```python
from build123d import *

# Parameters (mm, degrees)
F0_R        = 4.15
F1_DEPTH    = 2
F2_SIZE     = 1.99999
F3_T1_DEPTH = 51.7493718553


# Not quite as in the source:
# - a fillet or chamfer that OpenCascade refuses, or shapes differently, is made with other operations: its cross-section is extruded or revolved along the edge and cut away or added
# - a fillet or chamfer is up to 0.001 mm smaller than in the source, because OpenCascade refuses the exact size


with BuildPart() as f1:
    # F0 (on Front) → F1 (new body)
    with BuildSketch(Plane.XZ):
        Polygon((87.85, 18), (0, 18), (0, -18), (87.85, -18), (87.85, -9), (105.35, -9), (110.85, -1.42), (110.85, 1.42), (105.35, 9), (87.85, 9), align=None)
        with Locations((12, 0)):
            Circle(F0_R, mode=Mode.SUBTRACT)
        with Locations((28.5, 0)):
            Circle(F0_R, mode=Mode.SUBTRACT)
        Polygon((91.1, 5.5), (91.1, 3), (84.35, 3), (84.35, -3), (91.1, -3), (91.1, -5.5), (81.85, -5.5), (81.85, 5.5), align=None, mode=Mode.SUBTRACT)
    extrude(amount=F1_DEPTH)

    # F2 (size 2 in the source; OpenCascade refuses exactly that, so slightly less here)
    f2_edges = [f1.edges().sort_by_distance(p)[0] for p in [
        (7.85, -2, 0),
        (24.35, -2, 0),
    ]]
    chamfer(f2_edges, length=F2_SIZE)

    # F3: fillet of radius 10 on 2 edges, made by hand

    # F3_s2 → F3_t1 (cut)
    with BuildSketch(Plane.XZ.offset(-24.8746859277)):
        with BuildLine():
            ThreePointArc((77.9001256289, 18), (84.6083295614, 15.4161984871), (87.85, 9))
            Line((87.85, 9), (87.85, 18))
            Line((87.85, 18), (77.9001256289, 18))
        make_face()
        with BuildLine():
            ThreePointArc((77.9001256289, -18), (84.6083295614, -15.4161984871), (87.85, -9))
            Line((87.85, -9), (87.85, -18))
            Line((87.85, -18), (77.9001256289, -18))
        make_face()
    extrude(amount=F3_T1_DEPTH, mode=Mode.SUBTRACT)


solid = f1.part
```
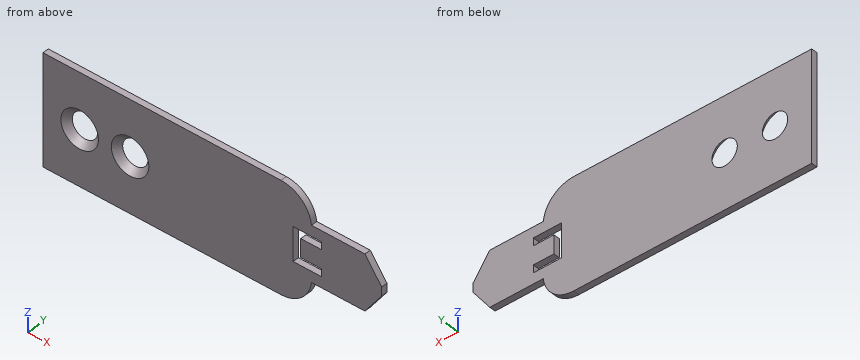
Here's how the part is built. I have some questions about the finished solid (model axes, mm). Coordinates: 2 decimals unless noted, no trailing zeros. Loops run counter-clockwise (first coordinate to the right, second up) from the corner with the lowest first, then second, coordinate; pieces in that order, holes last. Notation, with made-up numbers: (25, 30) - (58, 30) arc R21 ccw to (58, 36) - close; hole circle Ø3 at (48, 73). An arc over 180 degrees is marked (long way). Return JSON: item names as keys, results as strings. Group by question number.
Item 1: I need wall thicknesses on line 1 (X direction, y = -1.7, z = -1.5); line 2 (Z direction, x = 86.5, y = -1.1); line 3 (X direction, y = -1.9, z = 4.5). Which ranges of each line are inside material? Lowest first, please. Write a range as from..to.
Item 2: If we section it at B-B on z = 0: State how many separate pieces and enclosed holes the cut face has, and give its area (4 significant figures).
Item 3: Will these pins go through, and if not, where does the flat tip stop? P1, Ø6.5, axis at x = 12, z = 0, coming from the +Y side; P2, Ø1, axis at x = 87.5, y = -0.5, coming from the +Z side; P3, Ø1, axis at x = 98.5, y = -1, coming from the -Z side; P4, Ø1, axis at x = 51.5, z = -14, coming from the +Y side.
Item 4: If we section it at D-D on x = 93: Write out the boundary of the cut face in (y, z).
Item 5: If we section it at A-A on y = -1: Write out the boundary of the cut face in (x, z).
Calculated:
{
 "1": {"line 1": "x = 0..6.35, 17.65..22.85, 34.15..81.85, 84.35..110.79", "line 2": "z = -13.1..-5.5, -3..3, 5.5..13.1", "line 3": "x = 0..7.96, 16.04..24.46, 32.54..81.85, 91.1..108.62"},
 "2": {"separate pieces": "4", "enclosed holes": "0", "area": "175.5 mm^2"},
 "3": {"P1": "passes through", "P2": "stops at z = 12.15", "P3": "stops at z = -9", "P4": "stops at y = 0"},
 "4": {"outline": "(-2, -9) - (0, -9) - (0, 9) - (-2, 9) - close"},
 "5": {"outline": "(0, -18) - (77.9, -18) arc R10 ccw to (87.85, -9) - (105.35, -9) - (110.85, -1.42) - (110.85, 1.42) - (105.35, 9) - (87.85, 9) arc R10 ccw to (77.9, 18) - (0, 18) - close; hole circle Ø10.3 at (12, 0); hole circle Ø10.3 at (28.5, 0); hole (81.85, -5.5) - (91.1, -5.5) - (91.1, -3) - (84.35, -3) - (84.35, 3) - (91.1, 3) - (91.1, 5.5) - (81.85, 5.5) - close"}
}
